Check sheet for the modelled part. Datum: model origin and axes. Units: mm. Round coordinates to 2 decimals unless told otherwise and drop trailing zeros. Write each loop counter-clockwise with the first axis right and the second up, starting at its lowest first coordinate (ties: lowest second). Pieces come first, ordered by that corner, then holes. Notation, with made-up numbers: M -31.5,25 L 12.5,25 A21 cw 12.5,53 Z; hole C -24.5,-24.75 d4. An arc over 180 degrees is marked long. Put each result on its own line as item: value.
```python
from build123d import *

# Parameters (mm, degrees)
F3_SIZE = 3


# Not quite as in the source:
# - a fillet or chamfer that OpenCascade refuses, or shapes differently, is made with other operations: its cross-section is extruded or revolved along the edge and cut away or added


with BuildPart() as f1:
    # F0 (on Front) → F1 (revolve)
    with BuildSketch(Plane.XZ):
        Polygon((0, 8.25), (0, 0), (70, 0), (70, 4), (43, 4), (43, 7.6), (5, 7.6), (5, 8.25), align=None)
    revolve(axis=Axis((35, 0, 0), (1, 0, 0)))

    # F2: fillet of radius 5 on 1 edges, made by hand

    # F2_s1 → F2_t2 (revolve)
    with BuildSketch(Plane.XZ):
        with BuildLine():
            ThreePointArc((47.8, 4), (44.8, 5), (43, 7.6))
            Line((43, 7.6), (43, 4))
            Line((43, 4), (47.8, 4))
        make_face()
    revolve(axis=Axis((43, 0, 0), (1, 0, 0)))

    # F3
    f3_edges = [f1.edges().sort_by_distance(p)[0] for p in [
        (70, 0, -4),
    ]]
    chamfer(f3_edges, length=F3_SIZE)

    # F4: fillet of radius 8.1 on 1 edges, made by hand

    # F4_s1 → F4_t2 (revolve, cut)
    with BuildSketch(Plane.XZ):
        with BuildLine():
            ThreePointArc((5, 8.25), (1.3650167038, 5.2666852265), (0, 0.7666852265))
            Line((0, 0.7666852265), (0, 8.25))
            Line((0, 8.25), (5, 8.25))
        make_face()
    revolve(axis=Axis((0, 0, 0), (1, 0, 0)), mode=Mode.SUBTRACT)


solid = f1.part
```
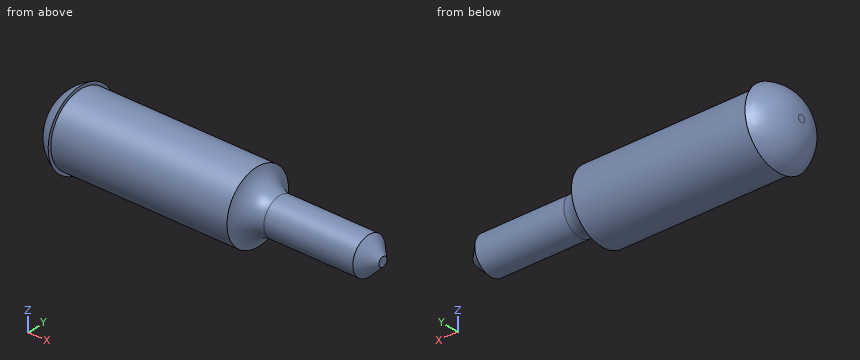
1. Scan lines: probe 1 along Y at (x, z) = (38, 2.75); probe 2 along Y at (x, z) = (31.5, 1.5). Record each from-to range of solid material in increasing order.
Computed values:
probe 1: y = -7.09 to 7.09
probe 2: y = -7.45 to 7.45
2. Depth check by flat-ended pin: pin 1 Ø1 at (x, y) = (19.5, 6) entering from +Z (3 decimals); pin 2 Ø1.5 at (y, z) = (1.5, -5.5) entering from -X; pin 3 Ø3 at (x, y) = (50.5, -2) entering from -Z. Enter the tip coordinate at first touch or a pass-through.
Computed values:
pin 1: stops at z = 5.245
pin 2: stops at x = 1.16
pin 3: stops at z = -3.97
3. Cross-section at B-B (x = 42). Enter the section's corners in (y, z), then the cut area to 3 significant figures.
Computed values:
outline: C 0,0 d15.2
area: 181 mm2
4. Cross-section at A-A (x = 51). Enter the section's corners in (y, z), then the cut area to 3 significant figures.
Computed values:
outline: C 0,0 d8
area: 50.3 mm2
